Read the model definition and answer for the solid it produces. Units are mm, in the model's axes. Face numbers are marked on the shaded views. A direction names the side the tool comes from. Give positions to 0.01 mm unless a question says otherwise; leave off trailing zeros. Order: outer loops, then holes, each group sorted by start corner. A loop starts at its lowest first (then second) coordinate and runs counter-clockwise, first axis right, second up. Notation, with made-up numbers: (82.25, 79.25) - (101.25, 79.25) arc R30 ccw to (101.25, 105.25) - close; hole circle Ø1 at (7, 33.25). An arc over 180 degrees is marked (long way). Write each question's results on one line, items separated by ' | '.
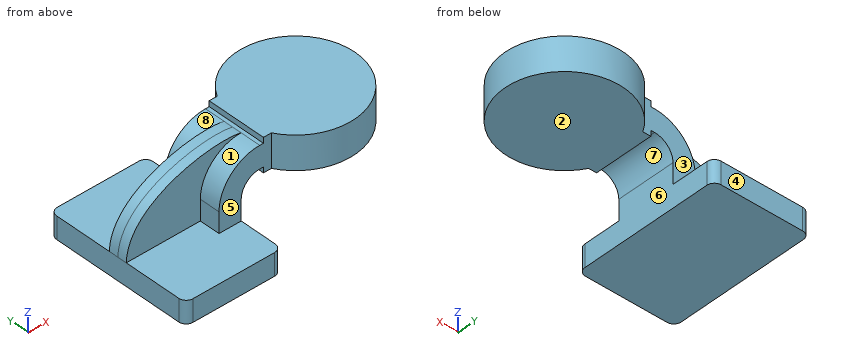
from build123d import *

# Parameters (mm, degrees)
F1_DEPTH = 63.5
F2_DEPTH = 25.4
F3_DEPTH = 7.9375
F5_R     = 6.35


with BuildPart() as f1:
    # F0 (on Front) → F1 (new body, symmetric)
    with BuildSketch(Plane.XZ):
        Polygon((22.225, 9.525), (-41.275, 9.525), (-41.275, -9.525), (41.275, -9.525), (41.275, 9.525), align=None)
    extrude(amount=F1_DEPTH, both=True)

    # F0 (on Front) → F2 (join, symmetric)
    with BuildSketch(Plane.XZ):
        with BuildLine():
            Line((22.225, 27.0002), (22.225, 9.525))
            Line((22.225, 9.525), (41.275, 9.525))
            Line((41.275, 9.525), (41.275, 27.0002))
            ThreePointArc((41.275, 27.0002), (45.92468, 38.22552), (57.15, 42.8752))
            Line((57.15, 42.8752), (60.325, 42.8752))
            Line((60.325, 42.8752), (60.325, 61.9252))
            Line((60.325, 61.9252), (57.15, 61.9252))
            ThreePointArc((57.15, 61.9252), (32.454296, 51.695904), (22.225, 27.0002))
        make_face()
        Polygon((60.325, 66.675), (60.325, 61.9252), (60.325, 42.8752), (60.325, 38.1), (111.125, 38.1), (111.125, 66.675), align=None)
    extrude(amount=F2_DEPTH, both=True)

    # F0 (on Front) → F3 (join, symmetric)
    with BuildSketch(Plane.XZ):
        with BuildLine():
            add(Edge.make_bspline(
                [(-41.275, 9.525), (-39.773323, 54.415304), (32.63097, 67.989412), (57.15, 61.9252)],
                knots=[0, 0, 0, 0, 111.504536, 111.504536, 111.504536, 111.504536], degree=3))
            Line((-41.275, 9.525), (22.225, 9.525))
            Line((22.225, 9.525), (22.225, 27.0002))
            ThreePointArc((22.225, 27.0002), (32.454296, 51.695904), (57.15, 61.9252))
        make_face()
    extrude(amount=F3_DEPTH, both=True)

    # F0 (on Front) → F4 (revolve)
    with BuildSketch(Plane.XZ):
        Polygon((60.325, 66.675), (60.325, 61.9252), (60.325, 42.8752), (60.325, 38.1), (111.125, 38.1), (111.125, 66.675), align=None)
    revolve(axis=Axis((111.125, 0, 52.3875), (0, 0, 1)))

    # F5
    f5_edges = [f1.edges().sort_by_distance(p)[0] for p in [
        (-41.275, -63.5, 0),
        (41.275, -63.5, 0),
        (41.275, 63.5, 0),
        (-41.275, 63.5, 0),
    ]]
    fillet(f5_edges, radius=F5_R)


solid = f1.part
(1) Each of these flat-tipped pins is pushed along its axis until it touches: pin 1 (8 mm diameter, centred on y = -43.5, z = 35, fed in from -X); pin 2 (16.5 mm diameter, centred on x = 3.5, y = -27, fed in from +Z) (3 decimals); pin 3 (16 mm diameter, centred on x = -3, z = 30, fed in from +Y); pin 4 (4 mm diameter, centred on y = 45.5, z = 10.5, fed in from -X) (3 decimals). Where does it stop, or does it pass through?
Conclusion:
pin 1: x = 81.09 | pin 2: z = 9.525 | pin 3: y = 7.94 | pin 4: x = -41.275
(2) Consider probe 1 along Z at (x, y) = (98.5, 7) (3 decimals); probe 2 along Y at (x, z) = (-24, 14); probe 3 along Z at (x, y) = (23.5, 48.5) (3 decimals). Determine where each line is inside the solid, lowest interval first. Write a range as [from, to].
Conclusion:
probe 1: [38.1, 66.675] | probe 2: [-7.94, 7.94] | probe 3: [-9.525, 9.525]
(3) Section B-B (y = -39) is taken. Give the vertices of the cut face in (x, z) (3 decimals), plus the area to 3 significant figures.
Conclusion:
outline: (-41.275, -9.525) - (41.275, -9.525) - (41.275, 9.525) - (-41.275, 9.525) - close; (78.573, 38.1) - (143.677, 38.1) - (143.677, 66.675) - (78.573, 66.675) - close | area: 3,430 mm^2
(4) The mould has two halves that part along X. Classify the marked faces 5, 6, 7 and 8: pulls with the +X half, pulls with the -X half, needs draft (parallel to the pull), parting line crosses it, or undercut.
Conclusion:
face 5: needs draft | face 6: pulls with the +X half | face 7: undercut | face 8: pulls with the -X half
(5) For the marked faces 1, 2, 3 and 4, determine the directions among +Z, -Z, +X, -X, +Y, -Y from which every point of the face is accessible in a straight line to the end or side of a thin tool.
Conclusion:
face 1: +Z, -X, -Y | face 2: -Z, +X, +Y, -Y | face 3: +Z, -X, +Y | face 4: +Z, -Z, +X, -X, +Y
(6) Section A-A (z = 3) is taken. Give the vertices of the cut face in (x, y) (3 decimals).
Conclusion:
outline: (-41.275, -57.15) arc R6.35 ccw to (-34.925, -63.5) - (34.925, -63.5) arc R6.35 ccw to (41.275, -57.15) - (41.275, 57.15) arc R6.35 ccw to (34.925, 63.5) - (-34.925, 63.5) arc R6.35 ccw to (-41.275, 57.15) - close
(7) Section C-C (y = 55) is taken. Give the vertices of the cut face in (x, z) (3 decimals).
Conclusion:
outline: (-41.275, -9.525) - (41.275, -9.525) - (41.275, 9.525) - (-41.275, 9.525) - close
(8) Section D-D (x = 73.5) is taken. Give the vertices of the cut face in (y, z) (3 decimals), plus the area to 3 significant figures.
Conclusion:
outline: (-34.132, 38.1) - (34.132, 38.1) - (34.132, 66.675) - (-34.132, 66.675) - close | area: 1,950 mm^2
